Source: CAD feature listing. Evaluate the final solid. Frame: model axes, mm. Give positions to 0.01 mm unless a question says otherwise; leave off trailing zeros. Order: outer loops, then holes, each group sorted by start corner. A loop starts at its lowest first (then second) coordinate and runs counter-clockwise, first axis right, second up. Notation, with made-up numbers: (-29, 5.5) -> (15, 5.5) arc R26 ccw to (15, 30.5) -> close; hole circle Ø7 at (0.5, 6.5). An arc over 180 degrees is marked (long way). Answer in a Markdown table with one row per item.
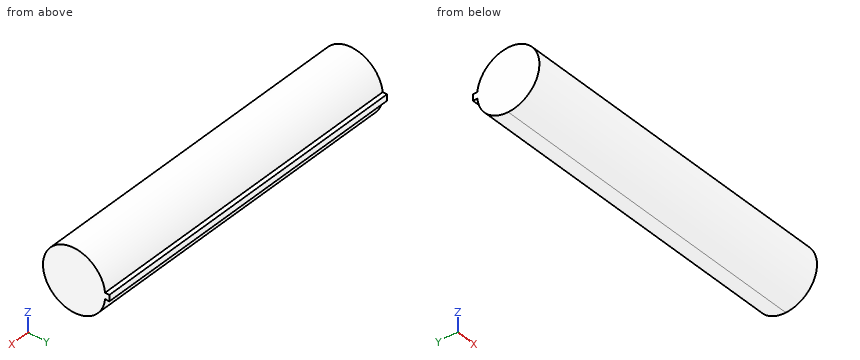
```python
from build123d import *

# Parameters (mm, degrees)
EXTRUDE_START   = -80
EXTRUDE_1_DEPTH = 160


with BuildPart() as part:
    # 草图1 → 凸台-拉伸1 (new body)
    with BuildSketch(Plane(origin=(0, 0, 0), x_dir=(0, 0, -1), z_dir=(1, 0, 0)).offset(EXTRUDE_START)):
        with BuildLine():
            Line((-1.5, 14.924811557), (-1.5, 0))
            Line((-1.5, 0), (1.5, 0))
            Line((1.5, 0), (1.5, 14.924811557))
            ThreePointArc((1.5, 14.924811557), (0, 15), (-1.5, 14.924811557))
        make_face()
        with BuildLine():
            Line((1.5, 0), (-1.5, 0))
            Line((-1.5, 0), (-1.5, 14.924811557))
            ThreePointArc((-1.5, 14.924811557), (-10.062305899, -11.124297731), (15, 0))
            ThreePointArc((15, 0), (11.124297731, 10.062305899), (1.5, 14.924811557))
            Line((1.5, 14.924811557), (1.5, 0))
        make_face()
        with BuildLine():
            Line((-1.5, 17), (-1.5, 14.924811557))
            ThreePointArc((-1.5, 14.924811557), (0, 15), (1.5, 14.924811557))
            Line((1.5, 14.924811557), (1.5, 17))
            Line((1.5, 17), (-1.5, 17))
        make_face()
    extrude(amount=EXTRUDE_1_DEPTH)


solid = part.part
```
(1) Section query A-A (x = -1). Return the cut outline in (y, z).
A:
| item | result |
|---|---|
| outline | (14.92, -1.5) -> (17, -1.5) -> (17, 1.5) -> (14.92, 1.5) arc R15 ccw (long way) to start |
(2) First-contact query: pin 1 Ø0.6 at (x, y) = (-33, 15.5) entering from +Z; pin 2 Ø5 at (x, y) = (-61, -6) entering from -Z; pin 3 Ø2 at (x, y) = (-24.5, 1.5) entering from +Z. Flat tips, straight axial feed; report the tip coordinate or a pass-through.
A:
| item | result |
|---|---|
| pin 1 | stops at z = 1.5 |
| pin 2 | stops at z = -14.59 |
| pin 3 | stops at z = 14.99 |
(3) Section query C-C (y = -5.5). Return the cut outline in (x, z), plus the area to 3 significant figures.
A:
| item | result |
|---|---|
| outline | (-80, -13.96) -> (80, -13.96) -> (80, 13.96) -> (-80, 13.96) -> close |
| area | 4,470 mm^2 |
(4) Ray query, probe 1 along Z at (x, y) = (14.5, 15); probe 2 along Y at (x, z) = (-50, 0); probe 3 along Y at (x, z) = (12.5, 10.5). Return the intervals inside material, ascending.
A:
| item | result |
|---|---|
| probe 1 | z = -1.5 to 1.5 |
| probe 2 | y = -15 to 17 |
| probe 3 | y = -10.71 to 10.71 |
(5) Section query B-B (z = -9). Return the cut outline in (x, y), plus the area to 3 significant figures.
A:
| item | result |
|---|---|
| outline | (-80, -12) -> (80, -12) -> (80, 12) -> (-80, 12) -> close |
| area | 3,840 mm^2 |
